Autodesk Inventor part; units mm, degrees
ref_plane "YZ Plane" through (0, 0, 0) normal (1, 0, 0) x (0, 1, 0)
ref_plane "XZ Plane" through (0, 0, 0) normal (0, 1, 0) x (-1, 0, 0)
ref_plane "XY Plane" through (0, 0, 0) normal (0, 0, 1) x (1, 0, 0)
sketch "スケッチ1" plane through (0, 0, 0) normal (0, 0, 1) x (1, 0, 0)
  line L0 (0, 0) -> (-15, 0)
  line L1 (-15, 0) -> (-15, -15)
  line L2 (-15, -15) -> (0, -15)
  line L3 (0, -15) -> (0, 0)
  line L4 (-13.8, -1.2) -> (-1.2, -1.2)
  line L5 (-1.2, -1.2) -> (-1.2, -13.8)
  line L6 (-1.2, -13.8) -> (-13.8, -13.8)
  line L7 (-13.8, -13.8) -> (-13.8, -1.2)
  dimension "d0" = 15
  dimension "d1" = 15
  dimension "d2" = 1.2
  dimension "d3" = 1.2
  dimension "d4" = 1.2
  dimension "d5" = 1.2
extrude "押し出し1" add sketch "スケッチ1" along normal blind 15
sketch "スケッチ2" plane through (0, -15, 0) normal (1, 0, 0) x (0, 0, -1)
  line L0 (-15, 0) -> (-15, 15)
  line L1 (0, 15) -> (-15, 15)
  point P0 (-7.5, 7.5)
  dimension "d8" = 7.5
  dimension "d9" = 7.5
hole "穴1" at (0, -7.5, 7.5) direction (-1, 0, 0) diameter 5 end through all
sketch "スケッチ3" plane through (-15, -15, 0) normal (0, -1, 0) x (1, 0, 0)
  line L0 (0, 0) -> (15, 0)
  line L1 (0, 0) -> (0, 15)
  point P0 (7.5, 7.5)
  dimension "d17" = 7.5
  dimension "d18" = 7.5
hole "穴2" at (-7.5, -15, 7.5) direction (0, 1, 0) diameter 7 end through all
equation "\"d3\" = d2"
equation "\"d4\" = d3"
equation "\"d5\" = d3"
properties part number "ロボットベース15x15x15" material "アルミニウム 6061"
The listing builds one solid part. Answer for the finished solid, in the listing's coordinates (mm). A direction names the side the tool comes from. Give positions to 0.01 mm unless a question says otherwise; leave off trailing zeros. Loops run counter-clockwise (first coordinate to the right, second up) from the corner with the lowest first, then second, coordinate; pieces in that order, holes last. Notation, with made-up numbers: M 86.25,27.25 L 137.25,27.25 A15 ccw 137.25,39.25 Z; hole C 15.5,83 d9. An arc over 180 degrees is marked long. One line per item, written item: value.
1. Find the intervals of material crossed by probe 1 along Y at (x, z) = (-11.5, 7.25); probe 2 along Z at (x, y) = (-0.15, -7.5), in increasing order.
Found:
probe 1: -15 to -13.8, -1.2 to 0
probe 2: 0 to 5, 10 to 15
2. For a pull along X with two mould halves and no side action, classify faces 1 (the face through (-9, -1.2, 4)), 2 (the face through (-15, -4, 7)), 3 (the face through (-4, 0, 9)) as pulls with the +X half, pulls with the -X half, needs draft (parallel to the pull), parting line crosses it, or undercut.
Found:
face 1: undercut
face 2: pulls with the -X half
face 3: needs draft
3. Section D-D on y = -13 is taken. Determine the outline of the cut face in (x, z).
Found:
outline: M -15,0 L -13.8,0 L -13.8,15 L -15,15 Z; M -1.2,0 L 0,0 L 0,15 L -1.2,15 Z
4. For faces 4 (the face through (-6, -13.8, 4)), 5 (the face through (-0.61, -5.06, 8.04)), determine the directions among +Z, -Z, +X, -X, +Y, -Y from which every point of the face is accessible in a straight line to the end or side of a thin tool.
Found:
face 4: +Z, -Z
face 5: +X, -X
5. Section B-B on z = 7.5 is taken. Determine the outline of the cut face in (x, y), plus the area to 3 significant figures.
Found:
outline: M -15,-15 L -11,-15 L -11,-13.8 L -13.8,-13.8 L -13.8,-10 L -15,-10 Z; M -15,-5 L -13.8,-5 L -13.8,-1.2 L -11,-1.2 L -11,0 L -15,0 Z; M -4,-15 L 0,-15 L 0,-10 L -1.2,-10 L -1.2,-13.8 L -4,-13.8 Z; M -4,-1.2 L -1.2,-1.2 L -1.2,-5 L 0,-5 L 0,0 L -4,0 Z
area: 37.4 mm^2
6. Section A-A on y = -7.5 is taken. Determine the outline of the cut face in (x, z), plus the area to 3 significant figures.
Found:
outline: M -15,0 L -13.8,0 L -13.8,5 L -15,5 Z; M -15,10 L -13.8,10 L -13.8,15 L -15,15 Z; M -1.2,0 L 0,0 L 0,5 L -1.2,5 Z; M -1.2,10 L 0,10 L 0,15 L -1.2,15 Z
area: 24.0 mm^2
7. Each of these flat-tipped pins is pushed along its axis until it touches: P1, Ø3, axis at y = -4, z = 7.5, coming from the +X side; P2, Ø4.5, axis at y = -7.5, z = 7.5, coming from the +X side. Where does it stop, or does it pass through?
Found:
P1: x = 0
P2: through
8. Section C-C on x = -7.5 is taken. Determine the outline of the cut face in (y, z).
Found:
outline: M -15,0 L -13.8,0 L -13.8,4 L -15,4 Z; M -15,11 L -13.8,11 L -13.8,15 L -15,15 Z; M -1.2,0 L 0,0 L 0,4 L -1.2,4 Z; M -1.2,11 L 0,11 L 0,15 L -1.2,15 Z
